Part model, mm, in its own coordinate system. Round coordinates to 2 decimals unless told otherwise and drop trailing zeros. Order: outer loops, then holes, each group sorted by start corner. A loop starts at its lowest first (then second) coordinate and runs counter-clockwise, first axis right, second up. Notation, with made-up numbers: (78, 19) - (127, 19) arc R6 cw to (127, 25) - close; hole circle Ø2 at (0.5, -27). An arc over 180 degrees is marked (long way). Return JSON: item names as keys, results as strings. Group by question number.
Item 1: Drop flat-ended pins along their axis: pin 1 (0.8 mm diameter, centred on x = -50.5, z = 3.5, fed in from +Y); pin 2 (4 mm diameter, centred on x = -44, y = -20, fed in from +Z); pin 3 (4 mm diameter, centred on x = 3, y = 49, fed in from +Z). Give the stop position or say it passes through.
Item 2: Probe probe 1 along Y at (x, z) = (0, 2.3) (3 decimals); probe 2 along Y at (x, z) = (0, 0.45) (3 decimals); probe 3 along Y at (x, z) = (-53.5, 1.5). List the from-to ranges inside material, lowest first.
Item 3: Saw through at C-C on x = -33. List the corners of the cut face in (y, z), and give its area (3 significant figures).
Item 4: Saw through at D-D on y = 32. List the corners of the cut face in (x, z), and give its area (3 significant figures).
Item 5: Two-plate mould, pull along X, no slides. Class faces 1 (the face through (14, -62, 5.5)), 2 (the face through (-13.955, -62.844, 3.979)), 3 (the face through (-27.207, -42.124, 3.24)): released by +X, released by -X, zero draft, split by the parting line, or undercut.
Item 6: Saw through at B-B on x = 0. State how many separate pieces and enclosed holes the cut face has, and give its area (4 significant figures).
```python
from build123d import *

# Parameters (mm, degrees)
F0_R      = 67
F1_DEPTH  = 2.5
F2_R      = 64.375
F2_R_2    = 62.625
F3_DEPTH  = 3
F4_R      = 4.75
F4_R_2    = 5.75
F4_R_3    = 2.1
F5_DEPTH  = 5.001
F6_R      = 5.75
F7_DEPTH  = 0.5
F6_R_2    = 6.75
F8_DEPTH  = 1
F2_R_3    = 58.875
F9_DEPTH  = 3
F10_R     = 6.75
F10_R_2   = 5.75
F11_DEPTH = 1
F13_W     = 5
F13_H     = 12
F14_DEPTH = 1.5
F15_COUNT = 6
F15_ANGLE = 150
F16_COUNT = 6
F16_ANGLE = 150
F17_DEPTH = 3


with BuildPart() as f1:
    # F0 (on Top) → F1 (new body, symmetric)
    with BuildSketch(Plane.XY):
        Circle(F0_R)
    extrude(amount=F1_DEPTH, both=True)

    # F2 (on face) → F3 (join)
    with BuildSketch(Plane.XY.offset(2.5)):
        Circle(F2_R)
        Circle(F2_R_2, mode=Mode.SUBTRACT)
    extrude(amount=F3_DEPTH)

    # F4 (on face) → F5 (cut, through all)
    with BuildSketch(Plane.XY.offset(2.5)):
        Circle(F4_R)
        with Locations((0, 18.75)):
            Circle(F4_R_2)
        with Locations((0, 46.25)):
            Circle(F4_R_2)
        with Locations((17.5, -8)):
            Circle(F4_R_3)
        with Locations((-17.5, -8)):
            Circle(F4_R_3)
    extrude(amount=-F5_DEPTH, mode=Mode.SUBTRACT)

    # F6 (on face) → F7 (cut)
    with BuildSketch(Plane.XY.offset(2.5)):
        Circle(F6_R)
    extrude(amount=-F7_DEPTH, mode=Mode.SUBTRACT)

    # F6 (on face) → F8 (cut)
    with BuildSketch(Plane.XY.offset(2.5)):
        with Locations((0, 18.75)):
            Circle(F6_R_2)
        with Locations((0, 46.25)):
            Circle(F6_R_2)
    extrude(amount=-F8_DEPTH, mode=Mode.SUBTRACT)

    # F2 (on face) → F9 (cut)
    with BuildSketch(Plane.XY.offset(2.5)):
        Circle(F2_R_2)
        Circle(F2_R_3, mode=Mode.SUBTRACT)
    extrude(amount=-F9_DEPTH, mode=Mode.SUBTRACT)

    # F10 (on face) → F11 (cut)
    with BuildSketch(Plane(origin=(0, 0, -2.5), x_dir=(1, 0, 0), z_dir=(0, 0, -1))):
        with Locations((0, -18.75)):
            Circle(F10_R)
        with Locations((0, -18.75)):
            Circle(F10_R_2, mode=Mode.SUBTRACT)
        with Locations((0, -46.25)):
            Circle(F10_R)
        with Locations((0, -46.25)):
            Circle(F10_R_2, mode=Mode.SUBTRACT)
    extrude(amount=-F11_DEPTH, mode=Mode.SUBTRACT)

    # F13 (on face) → F14 (join)
    with BuildSketch(Plane.XY.offset(2.5)):
        with Locations((0, -50)):
            Rectangle(F13_W, F13_H)
    f14 = extrude(amount=F14_DEPTH)

    # F15: F14 ×6 about axis
    f15_axis = Axis((0, 0, 2.5), (0, 0, 1))
    for i in range(1, F15_COUNT):
        add(f14.rotate(f15_axis, i * F15_ANGLE / (F15_COUNT - 1)))

    # F16: F14 ×6 about axis
    f16_axis = Axis((0, 0, 2.5), (0, 0, -1))
    for i in range(1, F16_COUNT):
        add(f14.rotate(f16_axis, i * F16_ANGLE / (F16_COUNT - 1)))

    # F6 (on face) → F17 (cut)
    with BuildSketch(Plane.XY.offset(2.5)):
        Polygon((-13.75, -10.1650635095), (-13.75, -5.8349364905), (-17.5, -3.6698729811), (-21.25, -5.8349364905), (-21.25, -10.1650635095), (-17.5, -12.3301270189), align=None)
        Polygon((21.25, -10.1650635095), (21.25, -5.8349364905), (17.5, -3.6698729811), (13.75, -5.8349364905), (13.75, -10.1650635095), (17.5, -12.3301270189), align=None)
    extrude(amount=-F17_DEPTH, mode=Mode.SUBTRACT)


solid = f1.part
```
Filled in:
{
 "1": {"pin 1": "stops at y = 40.42", "pin 2": "stops at z = 2.5", "pin 3": "stops at z = 1.5"},
 "2": {"probe 1": "y = -67 to -62.625, -58.875 to -5.75, 5.75 to 12, 25.5 to 39.5, 53 to 58.875, 62.625 to 67", "probe 2": "y = -67 to -62.625, -58.875 to -4.75, 4.75 to 13, 24.5 to 40.5, 52 to 58.875, 62.625 to 67", "probe 3": "y = -40.33 to -32.55, -24.58 to 24.58, 32.55 to 40.33"},
 "3": {"outline": "(-58.31, -2.5) - (58.31, -2.5) - (58.31, 2.5) - (55.27, 2.5) - (55.27, 5.5) - (53.22, 5.5) - (53.22, -0.5) - (48.76, -0.5) - (48.76, 2.5) - (-48.76, 2.5) - (-48.76, -0.5) - (-53.22, -0.5) - (-53.22, 5.5) - (-55.27, 5.5) - (-55.27, 2.5) - (-58.31, 2.5) - close", "area": "569 mm^2"},
 "4": {"outline": "(-58.86, -2.5) - (58.86, -2.5) - (58.86, 2.5) - (55.86, 2.5) - (55.86, 5.5) - (53.83, 5.5) - (53.83, -0.5) - (49.42, -0.5) - (49.42, 2.5) - (-49.42, 2.5) - (-49.42, -0.5) - (-53.83, -0.5) - (-53.83, 5.5) - (-55.86, 5.5) - (-55.86, 2.5) - (-58.86, 2.5) - close", "area": "574 mm^2"},
 "5": {"face 1": "zero draft", "face 2": "split by the parting line", "face 3": "undercut"},
 "6": {"separate pieces": "4", "enclosed holes": "0", "area": "504.5 mm^2"}
}
